Autodesk Inventor part; units mm, degrees
ref_plane "YZ Plane" through (0, 0, 0) normal (1, 0, 0) x (0, 1, 0)
ref_plane "XZ Plane" through (0, 0, 0) normal (0, 1, 0) x (-1, 0, 0)
ref_plane "XY Plane" through (0, 0, 0) normal (0, 0, 1) x (1, 0, 0)
sketch "スケッチ1" plane through (0, 0, 0) normal (0, 0, 1) x (1, 0, 0)
  line L0 (-50, 0) -> (50, 0) construction
  circle A0 centre (-50, 0) radius 4.05
  circle A1 centre (50, 0) radius 4.05
  line L1 (-50, 8.5) -> (43, 8.5)
  line L2 (-50, -8.5) -> (43, -8.5)
  arc A2 (-50, 8.5) -> (-50, -8.5) centre (-50, 0) ccw
  line L3 (43, -8.5) -> (50.119, -8.3992)
  line L4 (43, 8.5) -> (50.119, 8.3992)
  arc A3 (50.119, -8.3992) -> (50.119, 8.3992) centre (50, 0) ccw
  line L5 (9, -7.5) -> (38, -7.5) construction
  line L6 (38, -7.5) -> (38, -2.5) construction
  line L7 (38, -2.5) -> (9, -2.5) construction
  line L8 (9, -2.5) -> (9, -7.5) construction
  line L9 (9, -5) -> (38, -5) construction
  circle A4 centre (23.5, -5) radius 1.55
  circle A5 centre (11.5, -5) radius 1.55
  circle A6 centre (35.5, -5) radius 1.55
  line L10 (23.5, -5) -> (23.5, -2.5) construction
  line L11 (52.3191, 13) -> (22.3191, 13)
  line L12 (22.3191, 13) -> (12.3191, 8.5)
  line L13 (52.3191, 13) -> (57.3191, 4.122)
  point P0 (0, 0)
  point P1 (0, 0)
  point P2 (54.8534, 8.5)
  dimension "d0" = 100
  dimension "d1" = 8.1
  dimension "d2" = 8.5
  dimension "d8" = 8.1
  dimension "d9" = 7
  dimension "d10" = 8.4
  dimension "d12" = 5
  dimension "d13" = 29
  dimension "d14" = 3.1
  dimension "d15" = 2.5
  dimension "d17" = 13
  dimension "d19" = 10
  dimension "d20" = 30
  dimension "d25" = 12
  dimension "d26" = 5
  dimension "d45" = 1
extrude "押し出し1" add sketch "スケッチ1" along normal blind 2
fillet "フィレット1" radius 2 3 edges at (12.3191, 8.5, 1) (22.3191, 13, 1) (52.3191, 13, 1)
sketch "スケッチ2" plane through (0, 0, 0) normal (0, 0, -1) x (-1, 0, 0)
  circle A0 centre (-16.6795, 17.7128) radius 11.35 construction
  circle A1 centre (-16.6795, 17.7128) radius 11.55
  line L0 (-16.6795, 6.1628) -> (58.7547, 6.1628)
  line L1 (-16.6795, 17.7128) -> (-34, 27.7128) construction
  circle A2 centre (-50, 0) radius 4.05
  line L2 (-50, 0) -> (-34, 27.7128) construction
  line L3 (50, -8.5) -> (-43, -8.5)
  line L4 (-2.1795, 10.6628) -> (35.8205, 10.6628)
  line L5 (35.8205, 10.6628) -> (45.8205, 6.1628)
  line L6 (-2.1795, 10.6628) -> (-12.1795, 6.1628)
  circle A3 centre (50, 0) radius 4.05
  line L7 (58.7547, 6.1628) -> (-13.2236, 28.7337)
  arc A4 (50, -8.5) -> (50, 8.5) centre (50, 0) ccw
  point P0 (0, 0)
  dimension "d29" = 22.7
  dimension "d30" = 0.2
  dimension "d31" = 60
  dimension "d32" = 90
  dimension "d33" = 20
  dimension "d34" = 38
  dimension "d35" = 10
  dimension "d36" = 10
  dimension "d37" = 4.5
  dimension "d38" = 32
  dimension "d40" = 4.5
extrude "押し出し2" cut sketch "スケッチ2" against normal through all contours A1 | A1 L7 A4 L0 L5 L4 L6 | L7 L0 A4
fillet "フィレット2" radius 8 1 edges at (27.2242, 13, 1)
fillet "フィレット2" radius 2 2 edges at (12.1795, 6.1628, 1) (-45.8205, 6.1628, 1)
equation "\"d8\" = d1"
equation "\"d19\" = d18"
equation "\"d36\" = d35"
properties part number "リンク_メインフレーム_6_1" material "GFRP"
Model file for the job. Use its own axes, mm. A direction names the side the tool comes from. Round coordinates to 2 decimals unless told otherwise and drop trailing zeros. Order: outer loops, then holes, each group sorted by start corner. A loop starts at its lowest first (then second) coordinate and runs counter-clockwise, first axis right, second up. Notation, with made-up numbers: M -10,-16.75 L -3,-16.75 A21 cw -3,-0.75 Z; hole C -5.5,39 d8. An arc over 180 degrees is marked long. Write each question's results on one line, items separated by ' | '. Start each with the question number.
(1) Probe probe 1 along X at (y, z) = (-3, 1.2); probe 2 along Y at (x, z) = (11.5, 1.05); probe 3 along X at (y, z) = (-5.25, 1.65). List the from-to ranges inside material, lowest first. Write a range as from..to.
(2) Which spindle directions (+Z, -Z, +X, -X, +Y, -Y) get a long thin tool onto all of the face, cutting with end or side? Do faces 1 (the face through (21.57, 7.25, 0.99)), 2 (the face through (-1, 0, 2)), 3 (the face through (-51, 6.163, 1)). Say none if no direction does.
(3) Saw through at A-A, the plane x = 35.5. Give the cut face in (y, z).
(4) Saw through at B-B, the plane z = 0.6. Give the cut face in (x, y).
(5) Saw through at D-D, the plane x = -32.5. Give the cut face in (y, z), then the cut area to 3 significant figures.
(6) Drop flat-ended pins along their axis: pin 1 (0.6 mm diameter, centred on x = -49.5, z = 1, fed in from +Y); pin 2 (2.5 mm diameter, centred on x = 35.5, y = -5, fed in from -Z). Give the stop position or say it passes through.
(7) Saw through at C-C, the plane x = 15. Give the cut face in (y, z).
(8) Two-plate mould, pull along Y, no slides. Class faces 4 (the face through (9.353, 7.435, 0.986)), 5 (the face through (-4, -8.5, 1)), 6 (the face through (-53.214, 2.464, 0.986)): pulls with the +Y half, pulls with the -Y half, needs draft (parallel to the pull), parting line crosses it, or undercut.
Established:
1) probe 1: x = -57.95..-52.72, -47.28..47.28, 52.72..57.85 | probe 2: y = -8.5..-6.55, -3.45..6.47 | probe 3: x = -56.68..9.97, 13.03..21.97, 25.03..33.97, 37.03..56.56
2) face 1: +Z, -Z, +Y | face 2: +Z, +X, -X, +Y, -Y | face 3: +Z, -Z, -X, +Y
3) outline: M -8.5,0 L -6.55,0 L -6.55,2 L -8.5,2 Z; M -3.45,0 L 13,0 L 13,2 L -3.45,2 Z
4) outline: M -55.85,6.16 A8.5 ccw -50,-8.5 L 43,-8.5 L 50.12,-8.4 A8.4 ccw 57.32,4.12 L 52.89,11.98 A2 ccw 51.15,13 L 31.53,13 A8 ccw 25.45,10.2 A11.55 cw 16.68,6.16 L 12.61,6.16 A2 cw 11.79,6.34 L 6.99,8.5 L -40.63,8.5 L -45.43,6.34 A2 cw -46.25,6.16 Z; hole C -50,0 d8.1; hole C 11.5,-5 d3.1; hole C 23.5,-5 d3.1; hole C 35.5,-5 d3.1; hole C 50,0 d8.1
5) outline: M -8.5,0 L 8.5,0 L 8.5,2 L -8.5,2 Z | area: 34.0 mm^2
6) pin 1: stops at y = 6.16 | pin 2: passes through
7) outline: M -8.5,0 L 6.16,0 L 6.16,2 L -8.5,2 Z
8) face 4: pulls with the +Y half | face 5: pulls with the -Y half | face 6: undercut
